```python
from build123d import *

# Parameters (mm, degrees)
SKETCH_1_W          = 500
SKETCH_1_H          = 55
EXTRUDE_1_DEPTH     = 5
SKETCH_2_W          = 500
SKETCH_2_H          = 5
EXTRUDE_2_DEPTH     = 10
SKETCH_6_W          = 60
SKETCH_6_H          = 25
CUT_EXTRUDE_2_DEPTH = 365.413710539
SKETCH_7_W          = 18.6
SKETCH_7_H          = 3
EXTRUDE_5_DEPTH     = 380
SKETCH_8_R          = 3
CUT_EXTRUDE_3_DEPTH = 338.569517956


with BuildPart() as part:
    # 草图1 → 凸台-拉伸1 (new body)
    with BuildSketch(Plane.XY):
        with Locations((82.704402516, 120.419346185)):
            Rectangle(SKETCH_1_W, SKETCH_1_H)
    extrude(amount=EXTRUDE_1_DEPTH)

    # 草图2 → 凸台-拉伸2 (add)
    with BuildSketch(Plane(origin=(0, 0, 0), x_dir=(-1, 0, 0), z_dir=(0, 0, -1))):
        with Locations((-82.704402516, 115.419346185)):
            Rectangle(SKETCH_2_W, SKETCH_2_H)
    extrude(amount=EXTRUDE_2_DEPTH)

    # 草图6 → 切除-拉伸2 (cut, through all)
    with BuildSketch(Plane.XY.offset(5)):
        with Locations((302.704402516, 105.419346185)):
            Rectangle(SKETCH_6_W, SKETCH_6_H)
        with Locations((-137.295597484, 105.419346185)):
            Rectangle(SKETCH_6_W, SKETCH_6_H)
    extrude(amount=-CUT_EXTRUDE_2_DEPTH, mode=Mode.SUBTRACT)

    # 草图7 → 凸台-拉伸5 (add)
    with BuildSketch(Plane(origin=(272.704402516, 0, 0), x_dir=(0, 0, -1), z_dir=(1, 0, 0))):
        with Locations((-14.3, 94.419346185)):
            Rectangle(SKETCH_7_W, SKETCH_7_H)
    extrude(amount=-EXTRUDE_5_DEPTH)

    # 草图8 → 切除-拉伸3 (cut, through all)
    with BuildSketch(Plane(origin=(0, 95.919346185, 0), x_dir=(1, 0, 0), z_dir=(0, 1, 0))):
        with Locations(Location((-87.295597484, -12.6, 0), (0, 0, 270))):
            Circle(SKETCH_8_R)
        with Locations(Location((82.704402516, -12.6, 0), (0, 0, 270))):
            Circle(SKETCH_8_R)
        with Locations(Location((252.704402516, -12.6, 0), (0, 0, 270))):
            Circle(SKETCH_8_R)
    extrude(amount=-CUT_EXTRUDE_3_DEPTH, mode=Mode.SUBTRACT)


solid = part.part
```
Design review of the part built by this model. Coordinates are the model's own, in mm. A direction names the side the tool comes from. Coordinates: 2 decimals unless noted, no trailing zeros. Write each loop counter-clockwise with the first axis right and the second up, starting at its lowest first coordinate (ties: lowest second). Pieces come first, ordered by that corner, then holes.
1) Add section C-C (x = 284.5). Write out the cut boundary in (y, z).
2) Insertion check: pin 1 (15 mm diameter, centred on x = 13.5, y = 128, fed in from -Z); pin 2 (5 mm diameter, centred on x = 45.5, z = -7, fed in from +Y); pin 3 (22 mm diameter, centred on x = 167, y = 104.5, fed in from -Z); pin 4 (20 mm diameter, centred on y = 111.5, z = 13, fed in from -X). Each pin has a flat end and moves straight along its axis. Give the tip position at first contact, or say it passes through.
3) Add section B-B (y = 127.5). Write out the cut boundary in (x, z).
4) To check wall thickness, follow L1, parallel to X at y = 94, z = 12; L2, parallel to Y at x = 184.5, z = 14; L3, parallel to Z at x = 5, y = 125. State the ranges of each line that lie inside material, in increasing order.
5) Machinability: for faces 1 (the flat face through (85, 117.919, -5)), 2 (the flat face through (85.4, 95.919, 14.4)), 3 (the flat face through (80, 103, 0)), which of the approach directions +Z, -Z, +X, -X, +Y, -Y give a long, thin tool a straight path to every point of the face, cutting with its end or side? Answer none if there is none.
6) Add section A-A (x = 134.5). Write out the cut boundary in (y, z), plus the area to 3 significant figures.
Check result:
1. outline: (117.92, 0) - (147.92, 0) - (147.92, 5) - (117.92, 5) - close
2. pin 1: stops at z = 0
2. pin 2: stops at y = 117.92
2. pin 3: stops at z = -10
2. pin 4: stops at x = -107.3
3. outline: (-167.3, 0) - (332.7, 0) - (332.7, 5) - (-167.3, 5) - close
4. L1: x = -107.3 to -90.23, -84.36 to 79.77, 85.64 to 249.77, 255.64 to 272.7
4. L2: y = 92.92 to 95.92
4. L3: z = 0 to 5
5. face 1: -Z, +X, -X, +Y
5. face 2: +Z, +X, -X, +Y
5. face 3: -Z, +X, -X, -Y
6. outline: (92.92, 0) - (112.92, 0) - (112.92, -10) - (117.92, -10) - (117.92, 0) - (147.92, 0) - (147.92, 5) - (95.92, 5) - (95.92, 23.6) - (92.92, 23.6) - close
6. area: 381 mm2
